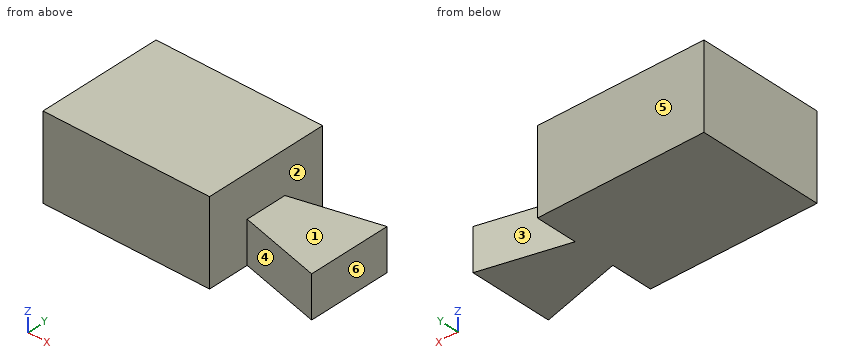
from build123d import *

# Parameters (mm, degrees)
F0_W     = 101.6
F0_H     = 50.8
F1_DEPTH = 76.2
F3_DEPTH = 25.4


with BuildPart() as f1:
    # F0 (on Front) → F1 (new body)
    with BuildSketch(Plane.XZ):
        with Locations((-20.575825, -13.165971)):
            Rectangle(F0_W, F0_H)
    extrude(amount=F1_DEPTH)

    # F2 (on face) → F3 (join)
    with BuildSketch(Plane(origin=(0, 0, -38.565971), x_dir=(1, 0, 0), z_dir=(0, 0, -1))):
        Polygon((81.024175, 63.5), (30.224175, 50.8), (30.224175, 25.4), (81.024175, 12.7), align=None)
    extrude(amount=-F3_DEPTH)


solid = f1.part
The model under review builds one solid part; all positions refer to its coordinate system, in mm. Face numbers are marked on the shaded views. A direction names the side the tool comes from. Round coordinates to 2 decimals unless told otherwise and drop trailing zeros. Order: outer loops, then holes, each group sorted by start corner. A loop starts at its lowest first (then second) coordinate and runs counter-clockwise, first axis right, second up. Notation, with made-up numbers: (-14, 40.5) - (5, 40.5) arc R16 cw to (5, 64.5) - close; hole circle Ø7 at (-32, 49). An arc over 180 degrees is marked (long way). Use one line per item in the form item = value.
Q1. Add section D-D on x = 54.5. Give the boundary of the cut face in (y, z), then the cut area to 3 significant figures.
Response values:
outline = (-56.87, -38.57) - (-19.33, -38.57) - (-19.33, -13.17) - (-56.87, -13.17) - close
area = 953 mm^2
Q2. Add section A-A on y = -17. Give the boundary of the cut face in (x, z).
Response values:
outline = (-71.38, -38.57) - (30.22, -38.57) - (30.22, 12.23) - (-71.38, 12.23) - close; (63.82, -38.57) - (81.02, -38.57) - (81.02, -13.17) - (63.82, -13.17) - close
Q3. Add section C-C on y = -30.5. Give the boundary of the cut face in (x, z).
Response values:
outline = (-71.38, -38.57) - (81.02, -38.57) - (81.02, -13.17) - (30.22, -13.17) - (30.22, 12.23) - (-71.38, 12.23) - close
Q4. Add section B-B on z = -26.5. Give the boundary of the cut face in (x, y), then the cut area to 3 significant figures.
Response values:
outline = (-71.38, -76.2) - (30.22, -76.2) - (30.22, -50.8) - (81.02, -63.5) - (81.02, -12.7) - (30.22, -25.4) - (30.22, 0) - (-71.38, 0) - close
area = 9,680 mm^2
Q5. To check wall thickness, follow line 1 (X direction, y = -63, z = -6.5); line 2 (Y direction, x = 31, z = -17.5). State the ranges of each line that lie inside material, in increasing order.
Response values:
line_1 = -71.38 to 30.22
line_2 = -50.99 to -25.21
Q6. Clearance check with flat-ended pins moving along their axes: P1, Ø4, axis at x = 38, y = -51, coming from the +Z side; P2, Ø12, axis at x = -42.5, z = -12, coming from the +Y side; P3, Ø12, axis at x = 61.5, z = -23, coming from the +Y side. State where each tip first meets the part, or that it passes through.
Response values:
P1 = -13.17
P2 = 0
P3 = -16.08
Q7. Tool access review of the marked faces 1, 2 and 3: name each direction out of +Z, -Z, +X, -X, +Y, -Y from which nothing blocks a thin tool from reaching the whole face with its end or side.
Response values:
face_1 = +Z, +X, +Y, -Y
face_2 = +Z
face_3 = +Z, -Z, +Y
Q8. Mouldability with a two-part tool opening along X and no side actions: class the marked faces 4, 5 and 6 as pulls with the +X half, pulls with the -X half, needs draft (parallel to the pull), parting line crosses it, or undercut.
Response values:
face_4 = undercut
face_5 = needs draft
face_6 = pulls with the +X half
